Design review of the part built by this model. Coordinates are the model's own, in mm. Face numbers are marked on the shaded views. A direction names the side the tool comes from. Round coordinates to 2 decimals unless told otherwise and drop trailing zeros. Loops run counter-clockwise (first coordinate to the right, second up) from the corner with the lowest first, then second, coordinate; pieces in that order, holes last. Notation, with made-up numbers: (50, 19) -> (107, 19) arc R22 cw to (107, 49) -> close; hole circle Ø7 at (8, -25.5). An arc over 180 degrees is marked (long way). Write each question's results on one line, items separated by ' | '. Start each with the question number.
from build123d import *

# Parameters (mm, degrees)
SKETCH2_W      = 74.93
SKETCH2_H      = 59.436
SKETCH2_W_2    = 68.58
SKETCH2_H_2    = 53.086
EXTRUDE1_DEPTH = 104.775
SKETCH4_W      = 1.5875
SKETCH4_H      = 11.4935
EXTRUDE2_DEPTH = 19.812
SKETCH13_W     = 68.58
SKETCH13_H     = 53.086
EXTRUDE4_DEPTH = 1.5875


with BuildPart() as part:
    # Sketch2 → Extrude1 (new body)
    with BuildSketch(Plane.XY):
        with Locations((37.465, 29.718)):
            Rectangle(SKETCH2_W, SKETCH2_H)
        with Locations((37.465, 29.718)):
            Rectangle(SKETCH2_W_2, SKETCH2_H_2, mode=Mode.SUBTRACT)
    extrude(amount=-EXTRUDE1_DEPTH)

    # Sketch4 → Extrude2 (cut)
    with BuildSketch(Plane(origin=(0, 59.436, 0), x_dir=(-1, 0, 0), z_dir=(0, 1, 0))):
        with Locations((-0.79375, -99.02825)):
            Rectangle(SKETCH4_W, SKETCH4_H)
        with Locations((-0.79375, -5.74675)):
            Rectangle(SKETCH4_W, SKETCH4_H)
        with Locations((-74.13625, -5.74675)):
            Rectangle(SKETCH4_W, SKETCH4_H)
        with Locations((-74.13625, -99.02825)):
            Rectangle(SKETCH4_W, SKETCH4_H)
    extrude(amount=-EXTRUDE2_DEPTH, mode=Mode.SUBTRACT)

    # Sketch13 → Extrude4 (add)
    with BuildSketch(Plane(origin=(0, 0, -104.775), x_dir=(-1, 0, 0), z_dir=(0, 0, -1))):
        with Locations((-37.465, 29.718)):
            Rectangle(SKETCH13_W, SKETCH13_H)
    extrude(amount=-EXTRUDE4_DEPTH)


solid = part.part
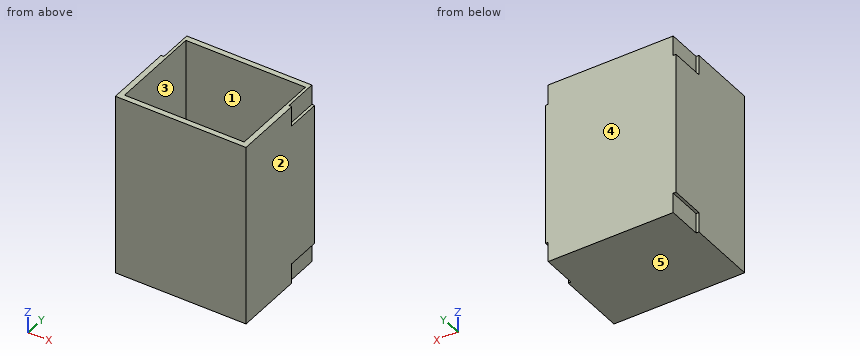
1) The part is to be moulded in two halves that separate along Y. For the marked faces 3, 4 and 5, say which applies: +Y half, -Y half, draft (parallel to the pull), parting line (faces both ways), or undercut.
2) Insertion check: pin 1 (3.5 mm diameter, centred on y = 50, z = -3, fed in from -X); pin 2 (1.7 mm diameter, centred on x = 0.5, y = 46.5, fed in from -Z); pin 3 (0.5 mm diameter, centred on x = 74.5, z = -3, fed in from +Y). Each pin has a flat end and moves straight along its axis. Give the tip position at first contact, or say it passes through.
3) Take a section at A-A (y = 6). Write out the cut boundary in (x, z) (1 decimal), plus the area to 3 significant figures.
4) Take a section at B-B (z = -51.5). Write out the cut boundary in (x, y) (3 decimals).
5) To check wall thickness, follow line 1 (X direction, y = 5.5, z = -32) (3 decimals); line 2 (Y direction, x = 12, z = -74.5) (3 decimals); line 3 (Z direction, x = 51, y = 55) (1 decimal). State the ranges of each line that lie inside material, in increasing order. Write a range as from..to.
6) For the marked faces 1 and 2, list the 3-axis set-ups (+Z, -Z, +X, -X, +Y, -Y) from which the entire face can be reached by the end or side of a thin tool; tool diameter is ignored.
7) Take a section at C-C (x = 59). Write out the cut boundary in (y, z) (1 decimal), plus the area to 3 significant figures.
Geometry check:
1) face 3: undercut | face 4: +Y half | face 5: draft
2) pin 1: stops at x = 1.59 | pin 2: stops at z = -93.28 | pin 3: stops at y = 39.62
3) outline: (0, -104.8) -> (74.9, -104.8) -> (74.9, 0) -> (71.8, 0) -> (71.8, -103.2) -> (3.2, -103.2) -> (3.2, 0) -> (0, 0) -> close | area: 774 mm^2
4) outline: (0, 0) -> (74.93, 0) -> (74.93, 59.436) -> (0, 59.436) -> close; hole (3.175, 3.175) -> (71.755, 3.175) -> (71.755, 56.261) -> (3.175, 56.261) -> close
5) line 1: x = 0..3.175, 71.755..74.93 | line 2: y = 0..3.175, 56.261..59.436 | line 3: z = -104.8..-103.2
6) face 1: +Z | face 2: +Z, -Z, +X, +Y, -Y
7) outline: (0, -104.8) -> (59.4, -104.8) -> (59.4, 0) -> (56.3, 0) -> (56.3, -103.2) -> (3.2, -103.2) -> (3.2, 0) -> (0, 0) -> close | area: 750 mm^2
